```python
from build123d import *

# Parameters (mm, degrees)
SKETCH2_R          = 4
CUT_EXTRUDE1_DEPTH = 40


with BuildPart() as part:
    # Sketch1 → Revolve1 (revolve)
    with BuildSketch(Plane(origin=(0, 0, 0), x_dir=(1, 0, 0), z_dir=(0, 1, 0)), mode=Mode.PRIVATE) as revolve1_sk:
        Polygon((6, 0), (-6, 0), (-6, 20), (-2, 20), (-2, 18.75), (2, 18.75), (2, 20), (6, 20), align=None)
    revolve(revolve1_sk.sketch.rotate(Axis((-28.819039277, 0, 0), (1, 0, 0)), 180), axis=Axis((-28.819039277, 0, 0), (1, 0, 0)))

    # Sketch2 → Cut-Extrude1 (cut)
    with BuildSketch(Plane.ZY.offset(6)):
        Circle(SKETCH2_R)
    extrude(amount=-CUT_EXTRUDE1_DEPTH, mode=Mode.SUBTRACT)


solid = part.part
```
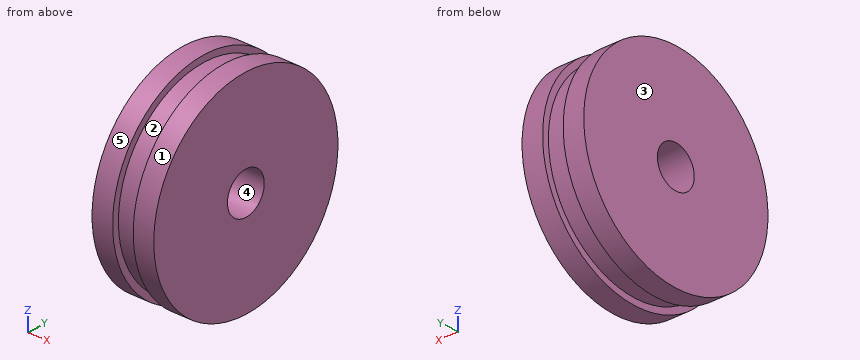
Check sheet for the modelled part. Datum: model origin and axes. Units: mm. Face numbers are marked on the shaded views. A direction names the side the tool comes from. Give positions to 0.01 mm unless a question says otherwise; leave off trailing zeros. Order: outer loops, then holes, each group sorted by start corner. A loop starts at its lowest first (then second) coordinate and runs counter-clockwise, first axis right, second up. Notation, with made-up numbers: M 71,-14.5 L 111,-14.5 A23 cw 111,21.5 Z; hole C -23,77 d1. An arc over 180 degrees is marked long. Answer in a Markdown table with one row per item.
1) Release check for a two-part mould opening along Z. For the marked faces 3, 4 and 5 record: +Z half, -Z half, draft (parallel to the pull), parting line (faces both ways), or undercut.
Filled sheet:
| item | result |
|---|---|
| face 3 | draft |
| face 4 | undercut |
| face 5 | parting line |
2) Gauge pin test, flat ends, axial feed: P1, Ø4, axis at x = -3, y = 13, coming from the -Z side; P2, Ø2, axis at x = -0.5, y = 4, coming from the -Z side; P3, Ø6, axis at x = 3.5, y = 4.5, coming from the +Z side. Record the tip position at first contact, or that the pin passes through.
Filled sheet:
| item | result |
|---|---|
| P1 | stops at z = -16.7 |
| P2 | stops at z = -18.51 |
| P3 | stops at z = 19.94 |
3) Cross-section at D-D, the plane x = -2.75. Enter the section's corners in (y, z).
Filled sheet:
| item | result |
|---|---|
| outline | C 0,0 d40; hole C 0,0 d8 |
4) Thickness scan on L1, parallel to Y at x = -1, z = 0; L2, parallel to Y at x = -3.5, z = 0; L3, parallel to X at y = -12.5, z = 14.5. Record the ranges inside material, lowest first. Write a range as [from, to].
Filled sheet:
| item | result |
|---|---|
| L1 | y = [-18.75, -4], [4, 18.75] |
| L2 | y = [-20, -4], [4, 20] |
| L3 | x = [-6, -2], [2, 6] |
5) Cross-section at C-C, the plane z = -16.5. Enter the section's corners in (x, y), plus the area to 3 significant figures.
Filled sheet:
| item | result |
|---|---|
| outline | M -6,-11.3 L -2,-11.3 L -2,-8.91 L 2,-8.91 L 2,-11.3 L 6,-11.3 L 6,11.3 L 2,11.3 L 2,8.91 L -2,8.91 L -2,11.3 L -6,11.3 Z |
| area | 252 mm2 |
6) Access from +Z, -Z, +X, -X, +Y, -Y to the whole of each face (thin tool, end or side, straight path). Record for the marked faces 1 and 2.
Filled sheet:
| item | result |
|---|---|
| face 1 | +X, -X |
| face 2 | none |
7) Cross-section at A-A, the plane y = 0. Enter the section's corners in (x, z), plus the area to 3 significant figures.
Filled sheet:
| item | result |
|---|---|
| outline | M -6,-20 L -2,-20 L -2,-18.75 L 2,-18.75 L 2,-20 L 6,-20 L 6,-4 L -6,-4 Z; M -6,4 L 6,4 L 6,20 L 2,20 L 2,18.75 L -2,18.75 L -2,20 L -6,20 Z |
| area | 374 mm2 |
